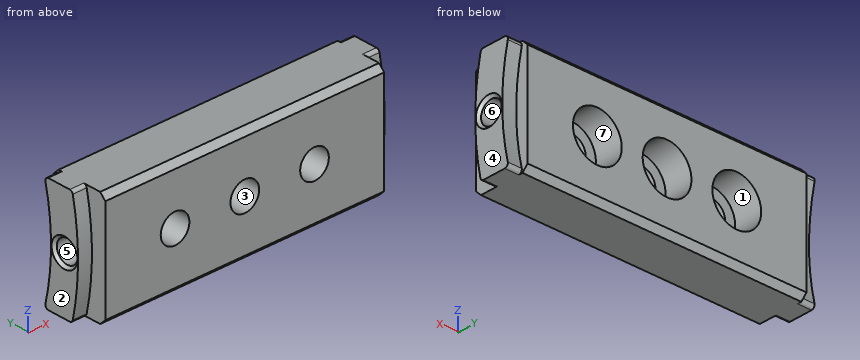
from build123d import *

# Parameters (mm, degrees)
SKETCH1_R                                        = 19.05
BOSS_EXTRUDE1_DEPTH                              = 12.7
CUT_EXTRUDE3_DEPTH                               = 30.784140075
SKETCH8_W                                        = 25.4
SKETCH8_H                                        = 4.850968343
CUT_EXTRUDE4_DEPTH                               = 30.784140075
SKETCH13_OUTSIDE_W                               = 49.628
SKETCH13_OUTSIDE_H                               = 37.157
SKETCH13_OUTSIDE_W_2                             = 25.4
SKETCH13_OUTSIDE_H_2                             = 25.629031657
CUT_EXTRUDE6_DEPTH                               = 27.940768363
SKETCH20_R                                       = 64.3382
CUT_EXTRUDE9_DEPTH                               = 3.175
BOSS_EXTRUDE4_DEPTH                              = 3.175
FILLET4_R                                        = 0.762
FILLET5_R                                        = 0.762
F_1_4_20_TAPPED_HOLE1_D                          = 5.1054
F_1_4_20_TAPPED_HOLE1_DEPTH                      = 9.525
F_1_4_20_TAPPED_HOLE1_CSINK_D                    = 6.35
F_1_4_20_TAPPED_HOLE1_CSINK_ANGLE                = 90
F_1_4_20_TAPPED_HOLE1_TIP                        = 1.533816902
SKETCH18_W                                       = 12.7
SKETCH18_H                                       = 9.525
BOSS_EXTRUDE3_DEPTH                              = 21.59
FILLET3_RADIUS                                   = 6.35
FILLET3_LENGTH                                   = 9.525
SKETCH19_R                                       = 3.175
CUT_EXTRUDE8_DEPTH                               = 42.79813026
SKETCH22_OUTSIDE_W                               = 38.286
SKETCH22_OUTSIDE_H                               = 59.325
SKETCH22_OUTSIDE_W_2                             = 25.4
SKETCH22_OUTSIDE_H_2                             = 19.685
CUT_EXTRUDE10_DEPTH                              = 41.042911819
BOSS_EXTRUDE5_DEPTH                              = 22.225
SKETCH26_OUTSIDE_W                               = 42.778
SKETCH26_OUTSIDE_H                               = 37.063
SKETCH26_OUTSIDE_W_2                             = 25.4
SKETCH26_OUTSIDE_H_2                             = 12.7
CUT_EXTRUDE11_DEPTH                              = 72.71846415
CHAMFER1_SIZE                                    = 1.27
CBORE_FOR_1_4_SOCKET_HEAD_CAP_SCREW1_D           = 6.5278
CBORE_FOR_1_4_SOCKET_HEAD_CAP_SCREW1_CBORE_D     = 11.1125
CBORE_FOR_1_4_SOCKET_HEAD_CAP_SCREW1_CBORE_DEPTH = 6.35


with BuildPart() as part:
    # Sketch1 → Boss-Extrude1 (new body)
    with BuildSketch(Plane(origin=(0, 0, 0), x_dir=(0, 0, -1), z_dir=(1, 0, 0))):
        Circle(SKETCH1_R)
    extrude(amount=BOSS_EXTRUDE1_DEPTH)

    # Sketch4 → Cut-Extrude3 (cut, through all)
    with BuildSketch(Plane(origin=(12.7, 0, 0), x_dir=(0, 0, -1), z_dir=(1, 0, 0))):
        with BuildLine():
            Line((-15.24, 21.59), (15.24, 21.59))
            Line((15.24, 21.59), (15.24, 11.43))
            ThreePointArc((15.24, 11.43), (0, 8.925760466), (-15.24, 11.43))
            Line((-15.24, 11.43), (-15.24, 21.59))
        make_face()
    extrude(amount=-CUT_EXTRUDE3_DEPTH, mode=Mode.SUBTRACT)

    # Sketch8 → Cut-Extrude4 (cut, through all)
    with BuildSketch(Plane.ZY):
        with Locations((0, -16.624515829)):
            Rectangle(SKETCH8_W, SKETCH8_H)
    extrude(amount=-CUT_EXTRUDE4_DEPTH, mode=Mode.SUBTRACT)

    # Sketch13 outside → Cut-Extrude6 (cut, through all)
    with BuildSketch(Plane(origin=(12.7, 0, 0), x_dir=(0, 0, -1), z_dir=(1, 0, 0))):
        with Locations((0, -1.3845)):
            Rectangle(SKETCH13_OUTSIDE_W, SKETCH13_OUTSIDE_H)
        with Locations((0, -1.384515828)):
            Rectangle(SKETCH13_OUTSIDE_W_2, SKETCH13_OUTSIDE_H_2, mode=Mode.SUBTRACT)
    extrude(amount=-CUT_EXTRUDE6_DEPTH, mode=Mode.SUBTRACT)

    # Sketch20 → Cut-Extrude9 (cut)
    with BuildSketch(Plane(origin=(12.7, 0, 0), x_dir=(0, 0, -1), z_dir=(1, 0, 0))):
        with Locations((0, 56.550760466)):
            Circle(SKETCH20_R)
    extrude(amount=-CUT_EXTRUDE9_DEPTH, mode=Mode.SUBTRACT)

    # Sketch21 → Boss-Extrude4 (add)
    with BuildSketch(Plane(origin=(9.525, 0, 0), x_dir=(0, 0, -1), z_dir=(1, 0, 0))):
        with BuildLine():
            Line((-12.7, -0.029636663), (-12.7, 6.760741289))
            ThreePointArc((-12.7, 6.760741289), (0, 5.166560466), (12.7, 6.760741289))
            Line((12.7, 6.760741289), (12.7, -0.029636663))
            ThreePointArc((12.7, -0.029636663), (0, -1.437439534), (-12.7, -0.029636663))
        make_face()
    extrude(amount=BOSS_EXTRUDE4_DEPTH)

    # Fillet4
    fillet4_edges = [part.edges().sort_by_distance(p)[0] for p in [
        (11.1125, -0.029636663, 12.7),
        (11.1125, -0.029636663, -12.7),
        (11.1125, 6.760741289, -12.7),
        (11.1125, 6.760741289, 12.7),
    ]]
    fillet(fillet4_edges, radius=FILLET4_R)

    # Fillet5
    fillet5_edges = [part.edges().sort_by_distance(p)[0] for p in [
        (11.1125, -6.521531226, 12.7),
        (11.1125, -6.521531226, -12.7),
    ]]
    fillet(fillet5_edges, radius=FILLET5_R)

    # 1/4-20 Tapped Hole1
    with Locations(Plane(origin=(12.7, 0, 0), x_dir=(0, 0, -1), z_dir=(1, 0, 0))):
        with Locations((0, 1.864560466)):
            CounterSinkHole(F_1_4_20_TAPPED_HOLE1_D / 2, F_1_4_20_TAPPED_HOLE1_CSINK_D / 2, depth=F_1_4_20_TAPPED_HOLE1_DEPTH, counter_sink_angle=F_1_4_20_TAPPED_HOLE1_CSINK_ANGLE)
            with Locations((0, 0, -(F_1_4_20_TAPPED_HOLE1_DEPTH + F_1_4_20_TAPPED_HOLE1_TIP / 2))):  # 118° drill point
                Cone(0, F_1_4_20_TAPPED_HOLE1_D / 2, F_1_4_20_TAPPED_HOLE1_TIP, mode=Mode.SUBTRACT)

    # Sketch18 → Boss-Extrude3 (add)
    with BuildSketch(Plane.XZ.offset(14.199031657)):
        with Locations((6.35, 0)):
            Rectangle(SKETCH18_W, SKETCH18_H)
    extrude(amount=BOSS_EXTRUDE3_DEPTH)

    # Fillet3: full round fillet: the end face becomes a half cylinder, R = half its width
    fillet3_face = Plane((6.35, -35.789031657, 0), x_dir=(0, 0, -1), z_dir=(0, -1, 0))  # on the end face: x along it, z out of the body
    fillet3_slab = fillet3_face.offset(-FILLET3_RADIUS / 2) * Box(FILLET3_LENGTH, 2 * FILLET3_RADIUS, FILLET3_RADIUS, mode=Mode.PRIVATE)  # the body's end, R deep
    fillet3_round = Plane((6.35, -29.439031657, 0), x_dir=(0, -1, 0), z_dir=(0, 0, -1)) * Cylinder(FILLET3_RADIUS, FILLET3_LENGTH, mode=Mode.PRIVATE)  # its axis R under the face
    add(fillet3_slab - fillet3_round, mode=Mode.SUBTRACT)

    # Sketch19 → Cut-Extrude8 (cut, through all)
    with BuildSketch(Plane.XY.offset(4.7625)):
        with Locations((6.35, -29.439031657)):
            Circle(SKETCH19_R)
    extrude(amount=-CUT_EXTRUDE8_DEPTH, mode=Mode.SUBTRACT)

    # Sketch22 outside → Cut-Extrude10 (cut, through all)
    with BuildSketch(Plane(origin=(12.7, 0, 0), x_dir=(0, 0, -1), z_dir=(1, 0, 0))):
        with Locations((0, -12.5695)):
            Rectangle(SKETCH22_OUTSIDE_W, SKETCH22_OUTSIDE_H)
        with Locations((0, 0.3175)):
            Rectangle(SKETCH22_OUTSIDE_W_2, SKETCH22_OUTSIDE_H_2, mode=Mode.SUBTRACT)
    extrude(amount=-CUT_EXTRUDE10_DEPTH, mode=Mode.SUBTRACT)

    # Sketch23 → Boss-Extrude5 (add)
    with BuildSketch(Plane.ZY):
        with BuildLine():
            Line((-10.77209211, 10.16), (-12.7, 10.16))
            Line((-12.7, 10.16), (-12.7, -9.525))
            Line((-12.7, -9.525), (12.7, -9.525))
            Line((12.7, -9.525), (12.7, 10.16))
            Line((12.7, 10.16), (10.77209211, 10.16))
            ThreePointArc((10.77209211, 10.16), (0, 8.925760466), (-10.77209211, 10.16))
        make_face()
    extrude(amount=BOSS_EXTRUDE5_DEPTH)

    # Mirror1: part across plane


with BuildPart() as part_1:
    add(part.part)
    add(part.part.mirror(Plane(origin=(-22.225, 56.550760466, 0), x_dir=(0, 0, 1), z_dir=(-1, 0, 0))))

    # Sketch26 outside → Cut-Extrude11 (cut, through all)
    with BuildSketch(Plane.ZY.offset(57.15)):
        with Locations((0, 0.3175)):
            Rectangle(SKETCH26_OUTSIDE_W, SKETCH26_OUTSIDE_H)
        with Locations((0, 1.624726526)):
            Rectangle(SKETCH26_OUTSIDE_W_2, SKETCH26_OUTSIDE_H_2, mode=Mode.SUBTRACT)
    extrude(amount=-CUT_EXTRUDE11_DEPTH, mode=Mode.SUBTRACT)

    # Chamfer1
    chamfer1_edges = [part_1.edges().sort_by_distance(p)[0] for p in [
        (-22.225, 7.974726526, -12.7),
        (-22.225, 7.974726526, 12.7),
        (-22.225, -4.725273474, 12.7),
        (-22.225, -4.725273474, -12.7),
    ]]
    chamfer(chamfer1_edges, length=CHAMFER1_SIZE)

    # CBORE for 1/4 Socket Head Cap Screw1 (through all)
    with Locations(Plane(origin=(0, 7.974726526, 0), x_dir=(1, 0, 0), z_dir=(0, 1, 0))):
        with Locations((-22.225, 0), (-38.1, 0), (-6.35, 0)):
            CounterBoreHole(CBORE_FOR_1_4_SOCKET_HEAD_CAP_SCREW1_D / 2, CBORE_FOR_1_4_SOCKET_HEAD_CAP_SCREW1_CBORE_D / 2, CBORE_FOR_1_4_SOCKET_HEAD_CAP_SCREW1_CBORE_DEPTH)


solid = part_1.part
The listing builds one solid part. Answer for the finished solid, in the listing's coordinates (mm). Face numbers are marked on the shaded views. A direction names the side the tool comes from. Round coordinates to 2 decimals unless told otherwise and drop trailing zeros. Order: outer loops, then holes, each group sorted by start corner. A loop starts at its lowest first (then second) coordinate and runs counter-clockwise, first axis right, second up. Notation, with made-up numbers: (31.5, -7.5) -> (59.5, -7.5) arc R22 ccw to (59.5, 22.5) -> close; hole circle Ø10 at (-14.75, 45.5). An arc over 180 degrees is marked (long way). One line per item, written item: value.
Item 1: Find section B-B, the plane z = 4.5. Give the vertices of the cut face in (x, y) (3 decimals).
Taken from the geometry:
outline: (-57.15, -1.263) -> (-53.975, -1.263) -> (-53.975, -4.725) -> (9.525, -4.725) -> (9.525, -1.263) -> (12.7, -1.263) -> (12.7, 5.364) -> (9.525, 5.364) -> (9.525, 7.975) -> (-3.091, 7.975) -> (-3.091, 1.625) -> (-9.609, 1.625) -> (-9.609, 7.975) -> (-18.966, 7.975) -> (-18.966, 1.625) -> (-25.484, 1.625) -> (-25.484, 7.975) -> (-34.841, 7.975) -> (-34.841, 1.625) -> (-41.359, 1.625) -> (-41.359, 7.975) -> (-53.975, 7.975) -> (-53.975, 5.364) -> (-57.15, 5.364) -> close
Item 2: For a pull along X with two mould halves and no side action, classify the marked faces 1, 2, 3 and 4 as released by +X, released by -X, zero draft, split by the parting line, or undercut.
Taken from the geometry:
face 1: undercut
face 2: released by -X
face 3: undercut
face 4: released by +X
Item 3: Find section D-D, the plane z = -0.75. State how many separate pieces and enclosed holes the cut face has, then the cut area to 3 significant figures.
Taken from the geometry:
separate pieces: 4
enclosed holes: 0
area: 418 mm2
Item 4: Find section A-A, the plane x = -6.35. Give the vertices of the cut face in (y, z), then the cut area to 3 significant figures.
Taken from the geometry:
outline: (-4.73, -11.43) -> (-3.46, -12.7) -> (6.7, -12.7) -> (7.97, -11.43) -> (7.97, -5.56) -> (1.62, -5.56) -> (1.62, -3.26) -> (-4.73, -3.26) -> close; (-4.73, 3.26) -> (1.62, 3.26) -> (1.62, 5.56) -> (7.97, 5.56) -> (7.97, 11.43) -> (6.7, 12.7) -> (-3.46, 12.7) -> (-4.73, 11.43) -> close
area: 207 mm2
Item 5: Given P1, Ø1.6, axis at y = -2.5, z = 5.5, coming from the +X side (3 decimals); P2, Ø7.5, axis at x = -6.35, z = 0, coming from the +Y side; P3, Ø0.8, axis at y = 6, z = 2.5, coming from the -X side (3 decimals), each flat-ended and moving along its own axis, determine where each tip first touches the part or whether it passes through.
Taken from the geometry:
P1: stops at x = 9.525
P2: stops at y = 1.62
P3: stops at x = -53.975
Item 6: Find section C-C, the plane x = -49.5. Give the vertices of the cut face in (y, z).
Taken from the geometry:
outline: (-4.73, -11.43) -> (-3.46, -12.7) -> (6.7, -12.7) -> (7.97, -11.43) -> (7.97, 11.43) -> (6.7, 12.7) -> (-3.46, 12.7) -> (-4.73, 11.43) -> close; hole circle Ø5.11 at (1.86, 0)
Item 7: Straight lines are drawn through the part: L1, parallel to Z at x = -38.1, y = -2; L2, parallel to X at y = 4.25, z = 1.25; L3, parallel to Y at x = 7.75, z = 0. For each, find the intervals that lie inside material, in ascending order.
Taken from the geometry:
L1: z = -12.7 to -3.26, 3.26 to 12.7
L2: x = -56.67 to -43.51, -32.69 to -27.64, -16.81 to -11.76, -0.94 to 12.22
L3: y = -4.73 to -0.69, 4.42 to 7.97
Item 8: For the marked faces 5, 6 and 7, determine the directions among +Z, -Z, +X, -X, +Y, -Y from which every point of the face is accessible in a straight line to the end or side of a thin tool.
Taken from the geometry:
face 5: -X
face 6: +X
face 7: +Y
